Verification items for the finished model (mm, model axes). Coordinates: 2 decimals unless noted, no trailing zeros. Order: outer loops, then holes, each group sorted by start corner. A loop starts at its lowest first (then second) coordinate and runs counter-clockwise, first axis right, second up. Notation, with made-up numbers: (-22, 28) -> (-3, 28) arc R12 ccw to (-3, 46) -> close; hole circle Ø8 at (13, 66). An arc over 180 degrees is marked (long way). Write each question's results on one line, items separated by ' | '. Start each with the question number.
(1) Cross-section at A-A on y = 0. Enter the section's corners in (x, z).
(2) Cross-section at B-B on z = 20. Enter the section's corners in (x, y).
(3) Thickness scan on probe 1 along Y at (x, z) = (-57, 5.25); probe 2 along X at (y, z) = (-9, 19.5); probe 3 along X at (y, z) = (7, 10.5). Record the ranges inside material, lowest first. Write a range as [from, to].
(4) Draft check along X on faces 1 (the cylindrical face through (-70.477, 0.558, 12.522)), 2 (the flat face through (73, 13, 0)), 3 (the flat face through (240.661, 12, 13)), 4 (the cylindrical face through (199.55, 8.58, 12.52)). Enter one of: +X half, -X half, draft (parallel to the pull), parting line (faces both ways), or undercut.
```python
from build123d import *

# Parameters (mm, degrees)
F0_W     = 165.1
F0_H     = 19.05
F0_R     = 12.7
F1_DEPTH = 25.4


with BuildPart() as f1:
    # F0 (on Top) → F1 (new body)
    with BuildSketch(Plane.XY):
        with Locations((158.11099, 53.975)):
            Rectangle(F0_W, F0_H)
        Polygon((75.56099, 44.45), (-89.53901, 44.45), (-89.53901, 0), (-89.53901, -38.1), (-57.78901, -38.1), (75.56099, -38.1), align=None)
        with Locations((-57.78901, 0)):
            Circle(F0_R, mode=Mode.SUBTRACT)
        Polygon((240.66099, 44.45), (75.56099, 44.45), (75.56099, -38.1), (208.91099, -38.1), (240.66099, -38.1), (240.66099, 0), align=None)
        with Locations((208.91099, 0)):
            Circle(F0_R, mode=Mode.SUBTRACT)
        with Locations((-6.98901, 53.975)):
            Rectangle(F0_W, F0_H)
    extrude(amount=F1_DEPTH)


solid = f1.part
```
Results are:
1) outline: (-89.54, 0) -> (-70.49, 0) -> (-70.49, 25.4) -> (-89.54, 25.4) -> close; (-45.09, 0) -> (196.21, 0) -> (196.21, 25.4) -> (-45.09, 25.4) -> close; (221.61, 0) -> (240.66, 0) -> (240.66, 25.4) -> (221.61, 25.4) -> close
2) outline: (-89.54, -38.1) -> (240.66, -38.1) -> (240.66, 63.5) -> (-89.54, 63.5) -> close; hole circle Ø25.4 at (-57.79, 0); hole circle Ø25.4 at (208.91, 0)
3) probe 1: y = [-38.1, -12.68], [12.68, 63.5] | probe 2: x = [-89.54, -66.75], [-48.83, 199.95], [217.87, 240.66] | probe 3: x = [-89.54, -68.39], [-47.19, 198.31], [219.51, 240.66]
4) face 1: undercut | face 2: draft | face 3: +X half | face 4: undercut
